from build123d import *
from build123d.topology import SkipClean

# Parameters (mm, degrees)
ESBO_O1_W                = 36
ESBO_O1_H                = 54.4
ESBO_O1_W_2              = 34
ESBO_O1_H_2              = 52.4
RESSALTO_EXTRUS_O1_DEPTH = 17
ESBO_O2_W                = 34
ESBO_O2_H                = 52.4
RESSALTO_EXTRUS_O2_DEPTH = 0.1
ESBO_O3_W                = 7.5
ESBO_O3_H                = 3
CORTE_EXTRUS_O1_DEPTH    = 5.5
ESBO_O4_W                = 2.4
ESBO_O4_H                = 1.1
CORTE_EXTRUS_O2_DEPTH    = 5.5
ESBO_O5_W                = 3
ESBO_O5_H                = 5
ESBO_O5_R                = 0.55
RESSALTO_EXTRUS_O3_DEPTH = 0.9
ESBO_O7_W                = 10.6
ESBO_O7_H                = 5.7
CORTE_EXTRUS_O3_DEPTH    = 3
ESBO_O8_W                = 1
ESBO_O8_H                = 6.5
RESSALTO_EXTRUS_O4_DEPTH = 3
ESBO_O9_W                = 1
ESBO_O9_H                = 6.5
RESSALTO_EXTRUS_O5_DEPTH = 3
ESBO_O10_W               = 1
ESBO_O10_H               = 5.6
RESSALTO_EXTRUS_O6_DEPTH = 3
RESSALTO_EXTRUS_O7_START = 0.5
ESBO_O11_R               = 0.55
RESSALTO_EXTRUS_O7_DEPTH = 0.5
ESBO_O12_W               = 1
ESBO_O12_H               = 6
CORTE_EXTRUS_O4_DEPTH    = 40


with BuildPart() as part:
    # Esboço1 → Ressalto-extrusão1 (new body)
    with BuildSketch(Plane(origin=(0, 0, 0), x_dir=(1, 0, 0), z_dir=(0, 1, 0))):
        Rectangle(ESBO_O1_W, ESBO_O1_H)
        Rectangle(ESBO_O1_W_2, ESBO_O1_H_2, mode=Mode.SUBTRACT)
    extrude(amount=RESSALTO_EXTRUS_O1_DEPTH)

    # Esboço2 → Ressalto-extrusão2 (add)
    with BuildSketch(Plane(origin=(0, 0, 0), x_dir=(1, 0, 0), z_dir=(0, 1, 0))):
        Rectangle(ESBO_O2_W, ESBO_O2_H)
    extrude(amount=RESSALTO_EXTRUS_O2_DEPTH)

    # Esboço3 → Corte-extrusão1 (cut, symmetric)
    with BuildSketch(Plane.XY.offset(27.2)):
        with Locations((0, 12.9)):
            Rectangle(ESBO_O3_W, ESBO_O3_H)
    extrude(amount=CORTE_EXTRUS_O1_DEPTH, both=True, mode=Mode.SUBTRACT)

    # Esboço4 → Corte-extrusão2 (cut, symmetric)
    with BuildSketch(Plane.XY.offset(-26.2)):
        with Locations((0, 5.95)):
            Rectangle(ESBO_O4_W, ESBO_O4_H)
    extrude(amount=CORTE_EXTRUS_O2_DEPTH, both=True, mode=Mode.SUBTRACT)

    # Esboço5 → Ressalto-extrusão3 (add)
    # profile 1 of 4: a face of its own
    with BuildSketch(Plane(origin=(0, 0, 0), x_dir=(1, 0, 0), z_dir=(0, 1, 0))):
        with Locations((19.5, -24.7)):
            Rectangle(ESBO_O5_W, ESBO_O5_H)
        with Locations(Location((19.4, -24.55, 0), (0, 0, 270))):
            Circle(ESBO_O5_R, mode=Mode.SUBTRACT)
    # profile 2 of 4: a face of its own
    with BuildSketch(Plane(origin=(0, 0, 0), x_dir=(1, 0, 0), z_dir=(0, 1, 0))):
        with Locations((-19.5, -24.7)):
            Rectangle(ESBO_O5_W, ESBO_O5_H)
        with Locations(Location((-19.4, -24.55, 0), (0, 0, 270))):
            Circle(ESBO_O5_R, mode=Mode.SUBTRACT)
    # profile 3 of 4: a face of its own
    with BuildSketch(Plane(origin=(0, 0, 0), x_dir=(1, 0, 0), z_dir=(0, 1, 0))):
        with Locations((-19.5, 24.7)):
            Rectangle(ESBO_O5_W, ESBO_O5_H)
        with Locations(Location((-19.4, 24.55, 0), (0, 0, 270))):
            Circle(ESBO_O5_R, mode=Mode.SUBTRACT)
    # profile 4 of 4: a face of its own
    with BuildSketch(Plane(origin=(0, 0, 0), x_dir=(1, 0, 0), z_dir=(0, 1, 0))):
        with Locations((19.5, 24.7)):
            Rectangle(ESBO_O5_W, ESBO_O5_H)
        with Locations(Location((19.4, 24.55, 0), (0, 0, 270))):
            Circle(ESBO_O5_R, mode=Mode.SUBTRACT)
    extrude(amount=RESSALTO_EXTRUS_O3_DEPTH)

    # Esboço7 → Corte-extrusão3 (cut)
    with BuildSketch(Plane(origin=(18, 0, 0), x_dir=(0, 0, -1), z_dir=(1, 0, 0))):
        with Locations((0, 14.15)):
            Rectangle(ESBO_O7_W, ESBO_O7_H)
    extrude(amount=-CORTE_EXTRUS_O3_DEPTH, mode=Mode.SUBTRACT)

    # Esboço8 → Ressalto-extrusão4 (add)
    with BuildSketch(Plane.ZY.offset(-17)):
        with Locations((15.7, 13.75)):
            Rectangle(ESBO_O8_W, ESBO_O8_H)
        with Locations((21.2, 13.75)):
            Rectangle(ESBO_O8_W, ESBO_O8_H)
    extrude(amount=RESSALTO_EXTRUS_O4_DEPTH)

    # Esboço9 → Ressalto-extrusão5 (add)
    with BuildSketch(Plane(origin=(-17, 0, 0), x_dir=(0, 0, -1), z_dir=(1, 0, 0))):
        with Locations((-21.2, 13.75)):
            Rectangle(ESBO_O9_W, ESBO_O9_H)
        with Locations((-15.7, 13.75)):
            Rectangle(ESBO_O9_W, ESBO_O9_H)
    extrude(amount=RESSALTO_EXTRUS_O5_DEPTH)

    # Esboço10 → Ressalto-extrusão6 (add)
    with BuildSketch(Plane(origin=(0, 0, 26.2), x_dir=(-1, 0, 0), z_dir=(0, 0, -1))):
        with Locations((4.75, 14.2)):
            Rectangle(ESBO_O10_W, ESBO_O10_H)
        with Locations((-4.75, 14.2)):
            Rectangle(ESBO_O10_W, ESBO_O10_H)
    extrude(amount=RESSALTO_EXTRUS_O6_DEPTH)

    # Esboço11 → Ressalto-extrusão7 (add)
    with SkipClean():  # the faces are left unmerged after this step: merging them gives an invalid solid
        with BuildSketch(Plane.XZ.offset(RESSALTO_EXTRUS_O7_START)):
            Polygon((-18, 22.2), (-18, -22.2), (-21, -22.2), (-21, -27.2), (21, -27.2), (21, -22.2), (18, -22.2), (18, 22.2), (21, 22.2), (21, 27.2), (-21, 27.2), (-21, 22.2), align=None)
            with Locations(Location((19.4, -24.55, 0), (0, 0, 270))):
                Circle(ESBO_O11_R, mode=Mode.SUBTRACT)
            with Locations(Location((19.4, 24.55, 0), (0, 0, 270))):
                Circle(ESBO_O11_R, mode=Mode.SUBTRACT)
            with Locations(Location((-19.4, 24.55, 0), (0, 0, 270))):
                Circle(ESBO_O11_R, mode=Mode.SUBTRACT)
            with Locations(Location((-19.4, -24.55, 0), (0, 0, 270))):
                Circle(ESBO_O11_R, mode=Mode.SUBTRACT)
        extrude(amount=-RESSALTO_EXTRUS_O7_DEPTH)

    # Esboço12 → Corte-extrusão4 (cut)
    with SkipClean():  # the faces are left unmerged after this step: merging them gives an invalid solid
        with BuildSketch(Plane(origin=(18, 0, 0), x_dir=(0, 0, -1), z_dir=(1, 0, 0))):
            with Locations((22.2, 12.5)):
                Rectangle(ESBO_O12_W, ESBO_O12_H)
            with Locations((16.7, 12.5)):
                Rectangle(ESBO_O12_W, ESBO_O12_H)
        extrude(amount=-CORTE_EXTRUS_O4_DEPTH, mode=Mode.SUBTRACT)


solid = part.part
Verification items for the finished model (mm, model axes). A direction names the side the tool comes from. Coordinates: 2 decimals unless noted, no trailing zeros. Write each loop counter-clockwise with the first axis right and the second up, starting at its lowest first coordinate (ties: lowest second). Pieces come first, ordered by that corner, then holes. Notation, with made-up numbers: M 68.5,67 L 109.5,67 A19 ccw 109.5,103 Z; hole C 42.5,86 d3. An arc over 180 degrees is marked long. Use CSV: the item, a comma, the result in double quotes.
Q1. Mould release check, pull along Z, two halves, no side actions. Record for faces 1 (the flat face through (19.5, 0.9, -25.3)), 2 (the flat face through (0, 8, -27.2)), 3 (the flat face through (16, 14, 15.2)): pulls with the +Z half, pulls with the -Z half, needs draft (parallel to the pull), parting line crosses it, or undercut.
Computed values:
face 1,"needs draft"
face 2,"pulls with the -Z half"
face 3,"undercut"
Q2. Section check B-B, the plane x = -12.5. Enter the section's corners in (y, z).
Computed values:
outline,"M -0.5,-27.2 L 17,-27.2 L 17,-26.2 L 0.1,-26.2 L 0.1,26.2 L 17,26.2 L 17,27.2 L -0.5,27.2 Z"
Q3. Go/stop test with flat-tipped pins: P1, Ø3, axis at y = 6, z = -4.5, coming from the +X side; P2, Ø1, axis at x = 7.5, z = 7.5, coming from the +Y side; P3, Ø1.1, axis at y = 12.5, z = 15.5, coming from the -X side. Record where each tip stops, or that it passes through.
Computed values:
P1,"x = 18"
P2,"y = 0.1"
P3,"x = -18"
Q4. Section check D-D, the plane y = 13.75. State how many separate pieces and enclosed holes the cut face has, and give its area (3 significant figures).
Computed values:
separate pieces,"6"
enclosed holes,"0"
area,"173 mm²"
Q5. Section check A-A, the plane y = 7.25. Enter the section's corners in (x, z).
Computed values:
outline,"M -18,-27.2 L 18,-27.2 L 18,27.2 L -18,27.2 Z; hole M -17,-26.2 L 17,-26.2 L 17,26.2 L -17,26.2 Z"
Q6. Section check C-C, the plane z = -11. Enter the section's corners in (x, y).
Computed values:
outline,"M -18,-0.5 L 18,-0.5 L 18,17 L 17,17 L 17,0.1 L -17,0.1 L -17,17 L -18,17 Z"
Q7. Set-up check for faces 4 (the flat face through (-20, 0.9, 25)), 5 (the flat face through (21, 0, 25)), 6 (the flat face through (-16, 14, 20.7)): record each of +Z, -Z, +X, -X, +Y, -Y from which the full face is reachable in a straight line by a thin tool's end or side.
Computed values:
face 4,"+Z, -Z, -X, +Y"
face 5,"+Z, -Z, +X, +Y, -Y"
face 6,"+Y"
Q8. Thickness scan on line 1 along Z through (x, y) = (-19.4, 0.6); line 2 along X through (y, z) = (-0.35, 24.55); line 3 along X through (y, z) = (0.3, 24.55). Record the ranges inside material, lowest first. Write a range as [from, to].
Computed values:
line 1,"[-27.2, -25.1], [-24, -22.2], [22.2, 24], [25.1, 27.2]"
line 2,"[-21, -19.95], [-18.85, 18.85], [19.95, 21]"
line 3,"[-21, -19.95], [-18.85, -17], [17, 18.85], [19.95, 21]"
